Build history of the part. All positions in model axes, mm. A direction names the side the tool comes from. Round coordinates to 2 decimals unless told otherwise and drop trailing zeros. Write each loop counter-clockwise with the first axis right and the second up, starting at its lowest first coordinate (ties: lowest second). Pieces come first, ordered by that corner, then holes. Notation, with made-up numbers: (-5, -7.5) - (23, -7.5) arc R27 ccw to (23, 28.5) - close; hole circle Ø1 at (-0.75, 15). An arc over 180 degrees is marked (long way). One line per question, with ' | ' between items.
from build123d import *

# Parameters (mm, degrees)
F0_W      = 120
F0_H      = 100
F1_DEPTH  = 10
F2_T      = -2.5
F4_W      = 3
F4_H      = 95
F5_DEPTH  = 10
F6_W      = 15
F6_H      = 2.5
F7_DEPTH  = 15
F8_W      = 15
F8_H      = 2.5
F8_H_2    = 97.5
F9_DEPTH  = 2
F10_W     = 15
F10_H     = 5
F11_DEPTH = 25
F12_R     = 5.5
F13_DEPTH = 5
F4_W_2    = 2
F4_H_2    = 20
F14_DEPTH = 3


with BuildPart() as f1:
    # F0 (on Top) → F1 (new body)
    with BuildSketch(Plane.XY):
        Rectangle(F0_W, F0_H)
    extrude(amount=F1_DEPTH)

    # F2
    f2_openings = [f1.faces().sort_by_distance(p)[0] for p in [
        (0, 0, 10),
    ]]
    offset(amount=F2_T, openings=f2_openings)

    # F4 (on face) → F5 (cut)
    with BuildSketch(Plane.XY.offset(2.5)):
        with Locations((58.746465, 0)):
            Rectangle(F4_W, F4_H)
    extrude(amount=F5_DEPTH, mode=Mode.SUBTRACT)

    # F6 (on face) → F7 (join)
    with BuildSketch(Plane.XY.offset(10)):
        with Locations((0, -48.75)):
            Rectangle(F6_W, F6_H)
        with Locations((0, 48.75)):
            Rectangle(F6_W, F6_H)
    extrude(amount=F7_DEPTH)

    # F8 (on face) → F9 (join)
    with BuildSketch(Plane.XY.offset(25)):
        with Locations((0, -48.75)):
            Rectangle(F8_W, F8_H)
        with Locations((0, 1.25)):
            Rectangle(F8_W, F8_H_2)
    extrude(amount=F9_DEPTH)

    # F10 (on face) → F11 (join)
    with BuildSketch(Plane.XY.offset(27)):
        Rectangle(F10_W, F10_H)
    extrude(amount=F11_DEPTH)

    # F12 (on face) → F13 (cut, through all)
    with BuildSketch(Plane.XZ.offset(2.5)):
        with Locations((0, 44.5)):
            Circle(F12_R)
    extrude(amount=-F13_DEPTH, mode=Mode.SUBTRACT)

    # F4 (on face) → F14 (join)
    with BuildSketch(Plane.XY.offset(2.5)):
        with Locations((55.273231, 0)):
            Rectangle(F4_W_2, F4_H_2)
    extrude(amount=F14_DEPTH)


solid = f1.part
Q1. Which spindle directions (+Z, -Z, +X, -X, +Y, -Y) get a long thin tool onto all of the face, cutting with end or side? Do faces 1 (the flat face through (0, 2.5, 37)), 2 (the flat face through (33, 49, 10)), 3 (the flat face through (0, -26, 27)), 4 (the flat face through (0, 1, 25)), 5 (the flat face through (54.273, 0, 4)). Say none if no direction does.
Found:
face 1: +Z, +X, -X, +Y | face 2: +Z, +X, +Y, -Y | face 3: +Z, +X, -X, -Y | face 4: +X, -X | face 5: +Z
Q2. Pull direction Z, two halves, no side cores. Call faces 6 (the flat face through (-59, 0, 10)), 7 (the flat face through (-1, -50, 7)), 8 (the flat face through (-1, 1, 0)), 9 (the flat face through (0, -47.5, 9)): +Z half, -Z half, draft (parallel to the pull), parting line (faces both ways), or undercut.
Found:
face 6: +Z half | face 7: draft | face 8: -Z half | face 9: undercut
Q3. Drill centre lines: L1, parallel to Z at x = 0, y = -0.85; L2, parallel to Y at x = 38.5, z = 3.5; L3, parallel to Z at x = 2, y = 21.5. Where is each one in solid material? Low to high. Write a range as from..to.
Found:
L1: 0..2.5, 25..39, 50..52 | L2: -50..-47.5, 47.5..50 | L3: 0..2.5, 25..27
Q4. Saw through at C-C, the plane x = 0. List the corners of the cut face in (y, z).
Found:
outline: (-50, 0) - (50, 0) - (50, 27) - (2.5, 27) - (2.5, 39) - (-2.5, 39) - (-2.5, 27) - (-50, 27) - close; (-2.5, 50) - (2.5, 50) - (2.5, 52) - (-2.5, 52) - close; hole (-47.5, 2.5) - (47.5, 2.5) - (47.5, 25) - (-47.5, 25) - close
Q5. Drop flat-ended pins along their axis: pin 1 (2 mm diameter, centred on x = 43.5, y = 49, fed in from +Z); pin 2 (7 mm diameter, centred on x = 23, z = 14.5, fed in from -Y); pin 3 (0.6 mm diameter, centred on x = 55.5, y = -4.5, fed in from +Z); pin 4 (1 mm diameter, centred on x = -5.5, z = 37, fed in from +Y). Give the stop position or say it passes through.
Found:
pin 1: z = 10 | pin 2: through | pin 3: z = 5.5 | pin 4: y = 2.5
Q6. Saw through at D-D, the plane x = 49. List the corners of the cut face in (y, z), then the cut area to 4 significant figures.
Found:
outline: (-50, 0) - (50, 0) - (50, 10) - (47.5, 10) - (47.5, 2.5) - (-47.5, 2.5) - (-47.5, 10) - (-50, 10) - close | area: 287.5 mm^2
Q7. Saw through at B-B, the plane z = 18.5. List the corners of the cut face in (x, y), then the cut area to 3 significant figures.
Found:
outline: (-7.5, -50) - (7.5, -50) - (7.5, -47.5) - (-7.5, -47.5) - close; (-7.5, 47.5) - (7.5, 47.5) - (7.5, 50) - (-7.5, 50) - close | area: 75.0 mm^2
Q8. Saw through at A-A, the plane y = -24. List the corners of the cut face in (x, z), then the cut area to 3 significant figures.
Found:
outline: (-60, 0) - (60, 0) - (60, 2.5) - (-57.5, 2.5) - (-57.5, 10) - (-60, 10) - close; (-7.5, 25) - (7.5, 25) - (7.5, 27) - (-7.5, 27) - close | area: 349 mm^2
